Source: CAD feature listing. Evaluate the final solid. Frame: model axes, mm. A direction names the side the tool comes from. Coordinates: 2 decimals unless noted, no trailing zeros. Order: outer loops, then holes, each group sorted by start corner. A loop starts at its lowest first (then second) coordinate and runs counter-clockwise, first axis right, second up. Notation, with made-up numbers: (-5.5, -5.75) - (49.5, -5.75) arc R22 ccw to (49.5, 2.25) - close; hole circle Ø3 at (24, 75.25). An arc over 180 degrees is marked (long way). One line per question, with ' | ' between items.
from build123d import *

# Parameters (mm, degrees)
SKETCH1_W                = 14.95
SKETCH1_H                = 20.95
SKETCH1_W_2              = 11
SKETCH1_H_2              = 16
BOSS_EXTRUDE1_DEPTH      = 2
SKETCH2_W                = 12.55
SKETCH2_H                = 17.3
BOSS_EXTRUDE2_DEPTH      = 13.3
SKETCH3_W                = 6.2
SKETCH3_H                = 18.44
BOSS_EXTRUDE3_DEPTH      = 8.8
BOSS_EXTRUDE4_DEPTH      = 2.525
BOSS_EXTRUDE4_DEPTH_BACK = 2.5
BOSS_EXTRUDE5_DEPTH      = 7.14
SKETCH6_W                = 2.5
SKETCH6_H                = 2
BOSS_EXTRUDE6_DEPTH      = 1


with BuildPart() as part:
    # Sketch1 → Boss-Extrude1 (new body)
    with BuildSketch(Plane.XY):
        Rectangle(SKETCH1_W, SKETCH1_H)
        Rectangle(SKETCH1_W_2, SKETCH1_H_2, mode=Mode.SUBTRACT)
    extrude(amount=BOSS_EXTRUDE1_DEPTH)

    # Sketch2 → Boss-Extrude2 (add)
    with BuildSketch(Plane(origin=(0, 0, 0), x_dir=(-1, 0, 0), z_dir=(0, 0, -1))):
        Rectangle(SKETCH2_W, SKETCH2_H)
    extrude(amount=BOSS_EXTRUDE2_DEPTH)

    # Sketch3 → Boss-Extrude3 (add)
    with BuildSketch(Plane.ZY.offset(6.275)):
        with Locations((-10.2, 0)):
            Rectangle(SKETCH3_W, SKETCH3_H)
    extrude(amount=-BOSS_EXTRUDE3_DEPTH)

    # Sketch4 → Boss-Extrude4 (add, two sides)
    with BuildSketch(Plane(origin=(0, 0, 0), x_dir=(0, 0, -1), z_dir=(1, 0, 0))) as boss_extrude4_sk:
        Polygon((7.1, -9.22), (4, -10.65), (3.35, -10.65), (3.35, -10.3705), (2.7, -10.3705), (2.7, -10.23075), (2.05, -10.23075), (2.05, -10.091), (1.4, -10.091), (1.4, -9.95125), (0.75, -9.95125), (0.75, -9.8115), (0, -9.8115), (0, -9.22), (4, -10.08), (7.1, -8.65), align=None)
        Polygon((7.1, 9.22), (7.1, 8.65), (4, 10.08), (0, 9.22), (0, 9.8115), (0.75, 9.8115), (0.75, 9.95125), (1.4, 9.95125), (1.4, 10.091), (2.05, 10.091), (2.05, 10.23075), (2.7, 10.23075), (2.7, 10.3705), (3.35, 10.3705), (3.35, 10.65), (4, 10.65), align=None)
    extrude(amount=BOSS_EXTRUDE4_DEPTH)
    extrude(boss_extrude4_sk.sketch, amount=-BOSS_EXTRUDE4_DEPTH_BACK)

    # Sketch5 → Boss-Extrude5 (add)
    with BuildSketch(Plane(origin=(0, 0, -13.3), x_dir=(-1, 0, 0), z_dir=(0, 0, -1))):
        Polygon((0.5, 6.35), (-0.5, 6.35), (-0.5, -0.58), (-6, -0.58), (-6, -1.58), (-0.5, -1.58), (-0.5, -8.65), (0.5, -8.65), (0.5, -1.58), (6, -1.58), (6, -0.58), (0.5, -0.58), align=None)
    extrude(amount=BOSS_EXTRUDE5_DEPTH)

    # Sketch6 → Boss-Extrude6 (add)
    with BuildSketch(Plane(origin=(0, 0, -13.3), x_dir=(-1, 0, 0), z_dir=(0, 0, -1))):
        with Locations((2.232930788, -2.58)):
            Rectangle(SKETCH6_W, SKETCH6_H)
        with Locations((2.232930788, -7.58)):
            Rectangle(SKETCH6_W, SKETCH6_H)
        with Locations((-2.232930788, -7.58)):
            Rectangle(SKETCH6_W, SKETCH6_H)
        with Locations((-2.232930788, -2.58)):
            Rectangle(SKETCH6_W, SKETCH6_H)
        with Locations((4.275, 6.35)):
            Rectangle(SKETCH6_W, SKETCH6_H)
        with Locations((-4.275, 6.35)):
            Rectangle(SKETCH6_W, SKETCH6_H)
    extrude(amount=BOSS_EXTRUDE6_DEPTH)


solid = part.part
(1) Cut plane D-D (z = -6.5). Return the cut outline in (x, y) (3 decimals), and give its area (3 significant figures).
Taken from the geometry:
outline: (-6.275, -8.65) - (6.275, -8.65) - (6.275, 8.65) - (-6.275, 8.65) - close; (-2.5, -9.497) - (2.525, -9.497) - (2.525, -8.927) - (-2.5, -8.927) - close; (-2.5, 8.927) - (2.525, 8.927) - (2.525, 9.497) - (-2.5, 9.497) - close | area: 223 mm²
(2) Pull-direction query (Y, two-part tool) for faces 1 (the flat face through (0, 10.475, 1)), 2 (the flat face through (-0.023, 9.656, -2.028)), 3 (the flat face through (0, -10.475, 1)); classes: pulls with the +Y half, pulls with the -Y half, needs draft (parallel to the pull), parting line crosses it, or undercut.
Taken from the geometry:
face 1: pulls with the +Y half | face 2: undercut | face 3: pulls with the -Y half
(3) Cut plane A-A (z = -16). Return the cut outline in (x, y).
Taken from the geometry:
outline: (-6, -1.58) - (-0.5, -1.58) - (-0.5, -8.65) - (0.5, -8.65) - (0.5, -1.58) - (6, -1.58) - (6, -0.58) - (0.5, -0.58) - (0.5, 6.35) - (-0.5, 6.35) - (-0.5, -0.58) - (-6, -0.58) - close
(4) Cut plane B-B (y = 6.75). Return the cut outline in (x, z) (3 decimals).
Taken from the geometry:
outline: (-7.475, 0) - (-6.275, 0) - (-6.275, -13.3) - (-5.525, -13.3) - (-5.525, -14.3) - (-3.025, -14.3) - (-3.025, -13.3) - (3.025, -13.3) - (3.025, -14.3) - (5.525, -14.3) - (5.525, -13.3) - (6.275, -13.3) - (6.275, 0) - (7.475, 0) - (7.475, 2) - (5.5, 2) - (5.5, 0) - (-5.5, 0) - (-5.5, 2) - (-7.475, 2) - close
(5) Pin query (flat end, axial travel): P1, Ø2, axis at y = -3.5, z = -18.5, coming from the -X side; P2, Ø4.5, axis at x = 4.5, z = -16, coming from the -Y side; P3, Ø12, axis at y = -7, z = -12, coming from the +X side (3 decimals); P4, Ø6.5, axis at x = -1.5, y = 1.5, coming from the -Z side. Return the tip coordinate at first contact, or that it passes through.
Taken from the geometry:
P1: stops at x = -0.5 | P2: stops at y = -8.58 | P3: stops at x = 6.275 | P4: stops at z = -20.44
(6) Material intervals for L1, parallel to X at y = -8.5, z = -13.5; L2, parallel to Y at x = 1, z = -1.75; L3, parallel to Z at x = -6, y = -5, sorted ascending. Write a range as from..to.
Taken from the geometry:
L1: x = -3.48..-0.98, -0.5..0.5, 0.98..3.48 | L2: y = -10.09..-9.6, -8.65..8.65, 9.6..10.09 | L3: z = -13.3..2
(7) Set-up query: faces 4 (the flat face through (-6, -1, -17)), 5 (the flat face through (0.983, -8, -14)), 6 (the flat face through (2, -6.58, -14)), 7 (the flat face through (-2, -3.58, -14)). Return all of +Z, -Z, +X, -X, +Y, -Y with unobstructed straight access to the full face (end or side cutting, diameter ignored); none if empty.
Taken from the geometry:
face 4: -Z, -X, +Y, -Y | face 5: -Z, -Y | face 6: -Z, +X | face 7: -Z, -X
(8) Cut plane C-C (x = 5). Return the cut outline in (y, z) (3 decimals), and give its area (3 significant figures).
Taken from the geometry:
outline: (-10.475, 0) - (-8.65, 0) - (-8.65, -13.3) - (-1.58, -13.3) - (-1.58, -20.44) - (-0.58, -20.44) - (-0.58, -13.3) - (5.35, -13.3) - (5.35, -14.3) - (7.35, -14.3) - (7.35, -13.3) - (8.65, -13.3) - (8.65, 0) - (10.475, 0) - (10.475, 2) - (8, 2) - (8, 0) - (-8, 0) - (-8, 2) - (-10.475, 2) - close | area: 249 mm²
